The model under review builds one solid part; all positions refer to its coordinate system, in mm. Round coordinates to 2 decimals unless told otherwise and drop trailing zeros. Loops run counter-clockwise (first coordinate to the right, second up) from the corner with the lowest first, then second, coordinate; pieces in that order, holes last. Notation, with made-up numbers: M -18,79.5 L 16,79.5 A32 ccw 16,107.5 Z; hole C 20.5,-5 d8. An arc over 180 degrees is marked long. One line per question, with ' | ' between items.
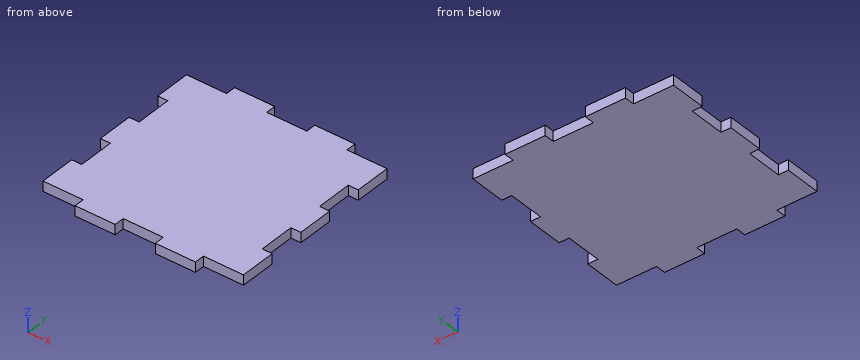
from build123d import *

# Parameters (mm, degrees)
ESQUISSE1_W             = 100
ESQUISSE1_H             = 90
BOSS_EXTRU_1_DEPTH      = 5
ESQUISSE2_OUTSIDE_W     = 128.926
ESQUISSE2_OUTSIDE_H     = 118.926
ENL_V_MAT_EXTRU_1_DEPTH = 5
ESQUISSE3_W             = 20
ESQUISSE3_H             = 5
BOSS_EXTRU_2_DEPTH      = 5


with BuildPart() as part:
    # Esquisse1 → Boss.-Extru.1 (new body)
    with BuildSketch(Plane.XY):
        with Locations((-50, -45)):
            Rectangle(ESQUISSE1_W, ESQUISSE1_H)
    extrude(amount=BOSS_EXTRU_1_DEPTH)

    # Esquisse2 outside → Enlèv. mat.-Extru.1 (cut)
    with BuildSketch(Plane.XY.offset(5)):
        with Locations((-50, -45)):
            Rectangle(ESQUISSE2_OUTSIDE_W, ESQUISSE2_OUTSIDE_H)
        Polygon((-100, 0), (-100, -18), (-95, -18), (-95, -36), (-100, -36), (-100, -54), (-95, -54), (-95, -72), (-100, -72), (-100, -90), (0, -90), (0, -72), (-5, -72), (-5, -54), (0, -54), (0, -36), (-5, -36), (-5, -18), (0, -18), (0, 0), align=None, mode=Mode.SUBTRACT)
    extrude(amount=-ENL_V_MAT_EXTRU_1_DEPTH, mode=Mode.SUBTRACT)

    # Esquisse3 → Boss.-Extru.2 (add)
    with BuildSketch(Plane.XY.offset(5)):
        with Locations((-70, 2.5)):
            Rectangle(ESQUISSE3_W, ESQUISSE3_H)
        with Locations((-30, 2.5)):
            Rectangle(ESQUISSE3_W, ESQUISSE3_H)
        with Locations((-70, -92.5)):
            Rectangle(ESQUISSE3_W, ESQUISSE3_H)
        with Locations((-30, -92.5)):
            Rectangle(ESQUISSE3_W, ESQUISSE3_H)
    extrude(amount=-BOSS_EXTRU_2_DEPTH)


solid = part.part
1) Insertion check: P1, Ø2.5, axis at x = -8.5, z = 2.5, coming from the +Y side; P2, Ø1.5, axis at y = 2.5, z = 2.5, coming from the +X side; P3, Ø2.5, axis at y = -91.5, z = 3.5, coming from the -X side. Each pin has a flat end and moves straight along its axis. Give the tip position at first contact, or say it passes through.
Output values:
P1: stops at y = 0 | P2: stops at x = -20 | P3: stops at x = -80
2) Add section A-A on x = -91. State the section outline as (y, z) points, then the cut area to 3 significant figures.
Output values:
outline: M -90,0 L 0,0 L 0,5 L -90,5 Z | area: 450 mm²
3) Add section B-B on y = -20. State the section outline as (x, z) points, then the cut area to 3 significant figures.
Output values:
outline: M -95,0 L -5,0 L -5,5 L -95,5 Z | area: 450 mm²
4) For line 1 (Y direction, x = -42, z = 4.4); line 2 (X direction, y = -20, z = 3.5), list the stretches that pass through material, from the lowest coordinate up.
Output values:
line 1: y = -90 to 0 | line 2: x = -95 to -5
